Verification items for the finished model (mm, model axes). Give positions to 0.01 mm unless a question says otherwise; leave off trailing zeros. Loops run counter-clockwise (first coordinate to the right, second up) from the corner with the lowest first, then second, coordinate; pieces in that order, holes last. Notation, with made-up numbers: (71, -17) -> (95, -17) arc R18 ccw to (95, 5) -> close; hole circle Ø8 at (-8.5, 76.5). An arc over 180 degrees is marked (long way). Answer in a Markdown table with one row per item. Add a question column.
Q1. Material ranges on probe 1 along X at (y, z) = (0.45, -3); probe 2 along Z at (x, y) = (16, 0.95); probe 3 along X at (y, z) = (1.4, 0), recorded low to high.
Q2. Section check B-B on y = 2.5. Give the number of separate pieces and of enclosed holes in the cut face, and give its area (3 significant figures).
Q3. Release check for a two-part mould opening along X. For faces 1 (the face through (-8, 0, -1)), 2 (the face through (22.08, 1.48, -15.54)) record: pulls with the +X half, pulls with the -X half, needs draft (parallel to the pull), parting line crosses it, or undercut.
Q4. Section check A-A on z = 0. Enter the section's corners in (x, y), and give its area (3 significant figures).
```python
from build123d import *

# Parameters (mm, degrees)
SKETCH4_R           = 39
BOSS_EXTRUDE1_DEPTH = 3
CUT_EXTRUDE1_DEPTH  = 3
SKETCH1_R           = 6.096
SKETCH1_R_2         = 1.7859375
CUT_EXTRUDE3_DEPTH  = 3
FILLET1_R           = 1


with BuildPart() as part:
    # Sketch4 → Boss-Extrude1 (new body)
    with BuildSketch(Plane(origin=(0, 0, 0), x_dir=(1, 0, 0), z_dir=(0, 1, 0))):
        with Locations(Location((0, 0, 0), (0, 0, 270))):
            Circle(SKETCH4_R)
    extrude(amount=BOSS_EXTRUDE1_DEPTH)

    # Sketch3 → Cut-Extrude1 (cut)
    with BuildSketch(Plane(origin=(0, 0, 0), x_dir=(1, 0, 0), z_dir=(0, 1, 0))):
        with BuildLine():
            Line((-0.65429081, -14.985723324), (-0.785148973, -17.982867988))
            ThreePointArc((-0.785148973, -17.982867988), (17.044742331, -5.785910375), (10.324375854, 14.744736797))
            Line((10.324375854, 14.744736797), (8.603646545, 12.287280664))
            ThreePointArc((8.603646545, 12.287280664), (14.203951942, -4.82159198), (-0.65429081, -14.985723324))
        make_face()
        with BuildLine():
            Line((1.439439783, -32.968591312), (1.570297945, -35.965735977))
            ThreePointArc((1.570297945, -35.965735977), (31.562163205, -17.315595681), (31.176914536, 18))
            Line((31.176914536, 18), (28.578838325, 16.5))
            ThreePointArc((28.578838325, 16.5), (28.931982938, -15.872629374), (1.439439783, -32.968591312))
        make_face()
        with BuildLine():
            Line((-1.570297945, 35.965735977), (-1.439439783, 32.968591312))
            ThreePointArc((-1.439439783, 32.968591312), (2.158303265, 32.929344467), (5.730389863, 32.498655849))
            Line((5.730389863, 32.498655849), (6.251334396, 35.453079108))
            ThreePointArc((6.251334396, 35.453079108), (2.354512652, 35.922921237), (-1.570297945, 35.965735977))
        make_face()
        with BuildLine():
            Line((12.31272516, 33.828934348), (11.28666473, 31.009856486))
            ThreePointArc((11.28666473, 31.009856486), (13.946402637, 29.908156972), (16.5, 28.578838325))
            Line((16.5, 28.578838325), (18, 31.176914536))
            ThreePointArc((18, 31.176914536), (15.214257423, 32.627080333), (12.31272516, 33.828934348))
        make_face()
        with BuildLine():
            Line((23.140353949, 27.577599952), (21.21199112, 25.279466623))
            ThreePointArc((21.21199112, 25.279466623), (23.334523779, 23.334523779), (25.279466623, 21.21199112))
            Line((25.279466623, 21.21199112), (27.577599952, 23.140353949))
            ThreePointArc((27.577599952, 23.140353949), (25.455844123, 25.455844123), (23.140353949, 27.577599952))
        make_face()
        with BuildLine():
            Line((1.308581621, 29.971446647), (1.177723459, 26.974301983))
            ThreePointArc((1.177723459, 26.974301983), (6.417519093, 26.226235885), (11.410693067, 24.47031025))
            Line((11.410693067, 24.47031025), (12.678547852, 27.189233611))
            ThreePointArc((12.678547852, 27.189233611), (7.13057677, 29.140262094), (1.308581621, 29.971446647))
        make_face()
        with BuildLine():
            Line((21.21199112, 21.214415682), (19.090792008, 19.092974114))
            ThreePointArc((19.090792008, 19.092974114), (22.116662678, 15.487195744), (24.47031025, 11.410693067))
            Line((24.47031025, 11.410693067), (27.189233611, 12.678547852))
            ThreePointArc((27.189233611, 12.678547852), (24.574069642, 17.207995271), (21.21199112, 21.214415682))
        make_face()
        with BuildLine():
            Line((19.659649063, 13.765834472), (17.20219293, 12.045105163))
            ThreePointArc((17.20219293, 12.045105163), (12.045105163, 17.20219293), (5.435199947, 20.284442352))
            Line((5.435199947, 20.284442352), (6.211657082, 23.182219831))
            ThreePointArc((6.211657082, 23.182219831), (13.765834472, 19.659649063), (19.659649063, 13.765834472))
        make_face()
    extrude(amount=CUT_EXTRUDE1_DEPTH, mode=Mode.SUBTRACT)

    # Sketch1 → Cut-Extrude3 (cut)
    with BuildSketch(Plane(origin=(0, 0, 0), x_dir=(1, 0, 0), z_dir=(0, 1, 0))):
        with Locations(Location((0, 0, 0), (0, 0, 270))):
            Circle(SKETCH1_R)
        with Locations(Location((6.914797213, 6.914797213, 0), (0, 0, 270))):
            Circle(SKETCH1_R_2)
        with Locations(Location((6.914797213, -6.914797213, 0), (0, 0, 270))):
            Circle(SKETCH1_R_2)
        with Locations(Location((-6.914797213, -6.914797213, 0), (0, 0, 270))):
            Circle(SKETCH1_R_2)
        with Locations(Location((-6.914797213, 6.914797213, 0), (0, 0, 270))):
            Circle(SKETCH1_R_2)
    extrude(amount=CUT_EXTRUDE3_DEPTH, mode=Mode.SUBTRACT)

    # Fillet1
    fillet1_edges = [part.edges().sort_by_distance(p)[0] for p in [
        (0, 0, -6.096),
        (0, 3, -6.096),
        (0, 0, -39),
        (0, 3, -39),
    ]]
    fillet(fillet1_edges, radius=FILLET1_R)


solid = part.part
```
Taken from the geometry:
| question | item | result |
|---|---|---|
| 1 | probe 1 | x = -38.72 to -5.5, 5.5 to 14.7, 17.75 to 32.86, 35.87 to 38.72 |
| 1 | probe 2 | z = -35.57 to -32.25, -28.86 to -17.89, -13.6 to -8.25, 8.25 to 28.86, 32.25 to 35.57 |
| 1 | probe 3 | x = -39 to -6.1, 6.1 to 15, 18 to 33, 36 to 39 |
| 2 | separate pieces | 1 |
| 2 | enclosed holes | 13 |
| 2 | area | 4,070 mm² |
| 3 | face 1 | needs draft |
| 3 | face 2 | undercut |
| 4 | outline | (-39, 1) arc R1 ccw to (-38, 0) -> (-7.1, 0) arc R1 ccw to (-6.1, 1) -> (-6.1, 2) arc R1 ccw to (-7.1, 3) -> (-38, 3) arc R1 ccw to (-39, 2) -> close; (6.1, 1) arc R1 ccw to (7.1, 0) -> (15, 0) -> (15, 3) -> (7.1, 3) arc R1 ccw to (6.1, 2) -> close; (18, 0) -> (33, 0) -> (33, 3) -> (18, 3) -> close; (36, 0) -> (38, 0) arc R1 ccw to (39, 1) -> (39, 2) arc R1 ccw to (38, 3) -> (36, 3) -> close |
| 4 | area | 178 mm² |
